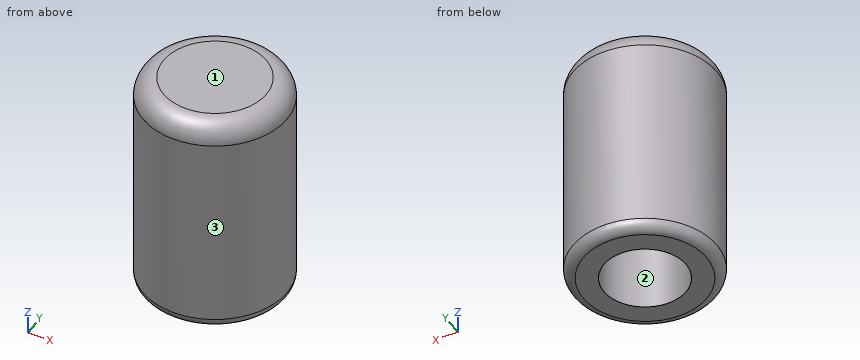
```python
from build123d import *

# Parameters (mm, degrees)
SKETCH1_R           = 7
SKETCH1_R_2         = 4
BOSS_EXTRUDE1_DEPTH = 20
SKETCH2_R           = 7
BOSS_EXTRUDE2_DEPTH = 2
FILLET1_R           = 2
FILLET2_R           = 1


with BuildPart() as part:
    # Sketch1 → Boss-Extrude1 (new body)
    with BuildSketch(Plane.XY):
        Circle(SKETCH1_R)
        Circle(SKETCH1_R_2, mode=Mode.SUBTRACT)
    extrude(amount=BOSS_EXTRUDE1_DEPTH)

    # Sketch2 → Boss-Extrude2 (add)
    with BuildSketch(Plane.XY.offset(20)):
        Circle(SKETCH2_R)
    extrude(amount=BOSS_EXTRUDE2_DEPTH)

    # Fillet1
    fillet1_edges = [part.edges().sort_by_distance(p)[0] for p in [
        (-7, 0, 22),
    ]]
    fillet(fillet1_edges, radius=FILLET1_R)

    # Fillet2
    fillet2_edges = [part.edges().sort_by_distance(p)[0] for p in [
        (-7, 0, 0),
    ]]
    fillet(fillet2_edges, radius=FILLET2_R)


solid = part.part
```
CAD build for the part. Positions are in the model's coordinates, mm. Face numbers are marked on the shaded views. Round coordinates to 2 decimals unless told otherwise and drop trailing zeros. Order: outer loops, then holes, each group sorted by start corner. A loop starts at its lowest first (then second) coordinate and runs counter-clockwise, first axis right, second up.
Q1. Drop flat-ended pins along their axis: pin 1 (2 mm diameter, centred on y = 2.5, z = 14, fed in from -X); pin 2 (2.5 mm diameter, centred on x = 1.5, y = -1, fed in from -Z); pin 3 (1 mm diameter, centred on y = -5, z = 18, fed in from +X). Give the stop position or say it passes through.
Q2. Slice it at C-C (z = 17.75). Write the cut outline in (x, y), and give its area (3 significant figures).
Q3. Wall check: L1, parallel to Y at x = 0, z = 10; L2, parallel to Z at x = 1.25, y = 0.25; L3, parallel to X at y = -2.25, z = 2.5. Give the ranges that are in metal, low to high.
Q4. Two-plate mould, pull along X, no slides. Class the marked faces 1, 2 and 3: pulls with the +X half, pulls with the -X half, needs draft (parallel to the pull), parting line crosses it, or undercut.
Q5. Slice it at A-A (y = 0). Write the cut outline in (x, z), and give its area (3 significant figures).
Results below:
1. pin 1: stops at x = -6.84
1. pin 2: stops at z = 20
1. pin 3: stops at x = 5.36
2. outline: circle Ø14 at (0, 0); hole circle Ø8 at (0, 0)
2. area: 104 mm2
3. L1: y = -7 to -4, 4 to 7
3. L2: z = 20 to 22
3. L3: x = -6.63 to -3.31, 3.31 to 6.63
4. face 1: needs draft
4. face 2: undercut
4. face 3: parting line crosses it
5. outline: (-7, 1) arc R1 ccw to (-6, 0) - (-4, 0) - (-4, 20) - (4, 20) - (4, 0) - (6, 0) arc R1 ccw to (7, 1) - (7, 20) arc R2 ccw to (5, 22) - (-5, 22) arc R2 ccw to (-7, 20) - close
5. area: 146 mm2
